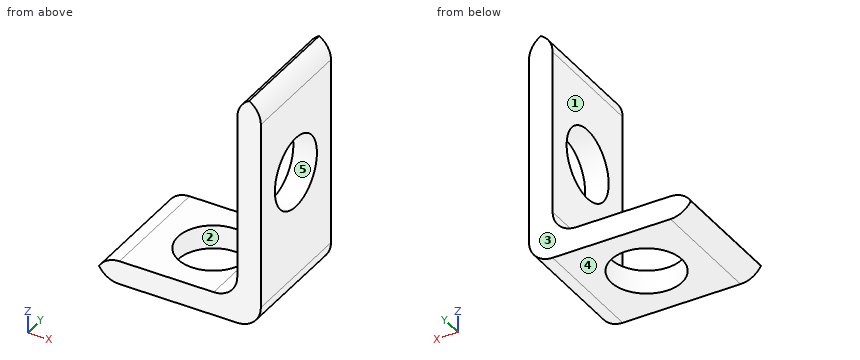
```python
from build123d import *

# Parameters (mm, degrees)
SKETCH1_W           = 7
SKETCH1_H           = 5
SKETCH1_R           = 1.5
BOSS_EXTRUDE1_DEPTH = 1
SKETCH2_W           = 1
SKETCH2_H           = 5
BOSS_EXTRUDE2_DEPTH = 9
SKETCH3_R           = 1.5
CUT_EXTRUDE1_DEPTH  = 1
FILLET1_R           = 1
FILLET2_R           = 1
FILLET3_R           = 1


# Some blends are built 0.0001 mm under size
with BuildPart() as part:
    # Sketch1 → Boss-Extrude1 (new body)
    with BuildSketch(Plane.XY):
        with Locations((3.5, 2.5)):
            Rectangle(SKETCH1_W, SKETCH1_H)
        with Locations((3.5, 2.5)):
            Circle(SKETCH1_R, mode=Mode.SUBTRACT)
    extrude(amount=BOSS_EXTRUDE1_DEPTH)

    # Sketch2 → Boss-Extrude2 (add)
    with BuildSketch(Plane.XY.offset(1)):
        with Locations((6.5, 2.5)):
            Rectangle(SKETCH2_W, SKETCH2_H)
    extrude(amount=BOSS_EXTRUDE2_DEPTH)

    # Sketch3 → Cut-Extrude1 (cut)
    with BuildSketch(Plane.ZY.offset(-6)):
        with Locations(Location((5.5, 2.5, 0), (0, 0, 270))):
            Circle(SKETCH3_R)
    extrude(amount=-CUT_EXTRUDE1_DEPTH, mode=Mode.SUBTRACT)

    # Fillet1
    fillet1_edges = [part.edges().sort_by_distance(p)[0] for p in [
        (6, 2.5, 1),
    ]]
    fillet(fillet1_edges, radius=FILLET1_R - 0.0001)  # a hair under: the kernel refuses the full size

    # Fillet2
    # the kernel refuses this fillet: 1 mm, written as the material it takes off along each edge
    with BuildSketch(Plane(origin=(7, -2.5, 10), x_dir=(-1, 0, 0), z_dir=(0, 1, 0)), Plane(origin=(0, 7.5, 0), x_dir=(0, 0, 1), z_dir=(0, -1, 0)), Plane(origin=(0, 7.5, 1), x_dir=(1, 0, 0), z_dir=(0, -1, 0))) as fillet2_piece_1:
        with BuildLine():
            CenterArc((FILLET2_R, -FILLET2_R), FILLET2_R, 90, 90)
            Line((0, -FILLET2_R), (0, 0))
            Line((0, 0), (FILLET2_R, 0))
        make_face()
    extrude(amount=10, mode=Mode.SUBTRACT)
    with BuildSketch(Plane(origin=(6, 7.5, 10), x_dir=(0, 0, -1), z_dir=(0, -1, 0))) as fillet2_piece_2:
        with BuildLine():
            CenterArc((FILLET2_R, FILLET2_R), FILLET2_R, 180, 90)
            Line((0, FILLET2_R), (0, 0))
            Line((0, 0), (FILLET2_R, 0))
        make_face()
    extrude(amount=10, mode=Mode.SUBTRACT)

    # Fillet3
    fillet3_edges = [part.edges().sort_by_distance(p)[0] for p in [
        (7, 2.5, 0),
    ]]
    fillet(fillet3_edges, radius=FILLET3_R)


solid = part.part
```
Build history of the part. All positions in model axes, mm. Face numbers are marked on the shaded views. A direction names the side the tool comes from. Round coordinates to 2 decimals unless told otherwise and drop trailing zeros. Loops run counter-clockwise (first coordinate to the right, second up) from the corner with the lowest first, then second, coordinate; pieces in that order, holes last. Notation, with made-up numbers: M -38.5,-3 L -15.5,-3 A25 cw -15.5,31 Z; hole C -11.75,62 d2. An arc over 180 degrees is marked long. Answer as CSV lines item,"result".
1. Cut at C-C on x = 3.5. Write the cut outline in (y, z).
Resolved:
outline,"M 0,0 L 1,0 L 1,1 L 0,1 Z; M 4,0 L 5,0 L 5,1 L 4,1 Z"
2. Cut at D-D on y = 0.8. Write the cut outline in (x, z).
Resolved:
outline,"M 0.13,0.5 A1 ccw 1,0 L 6,0 A1 ccw 7,1 L 7,9 A1 ccw 6.5,9.87 A1 ccw 6,9 L 6,2 A1 cw 5,1 L 1,1 A1 ccw Z"
3. Two-plate mould, pull along Y, no slides. Class the marked faces 3, 4 and 5: released by +Y, released by -Y, zero draft, split by the parting line, or undercut.
Resolved:
face 3,"released by +Y"
face 4,"zero draft"
face 5,"undercut"
4. Flat gauge pins, fed straight in: P1, Ø1.5, axis at y = 2.5, z = 8, coming from the -X side; P2, Ø1.8, axis at x = 3.5, y = 2.5, coming from the -Z side; P3, Ø3, axis at x = 5.5, z = 7, coming from the -Y side. Where does each tip first touch, or does it go through?
Resolved:
P1,"stops at x = 6"
P2,"passes through"
P3,"stops at y = 0"
5. Wall check: probe 1 along Y at (x, z) = (3.5, 0.7); probe 2 along X at (y, z) = (4.35, 3); probe 3 along Z at (x, y) = (1, 2.2). Give the ranges that are in metal, low to high. Write a range as [from, to].
Resolved:
probe 1,"y = [0, 1], [4, 5]"
probe 2,"x = [6, 7]"
probe 3,"z = [0, 1]"
6. 3-axis set-ups, long thin cutter, end or side, ignore diameter. For the marked faces 1 and 2: which of +Z, -Z, +X, -X, +Y, -Y reach the whole face in a straight line?
Resolved:
face 1,"+Z, -X, +Y, -Y"
face 2,"+Z, -Z"
7. Cut at A-A on z = 5.5. Write the cut outline in (x, y).
Resolved:
outline,"M 6,0 L 7,0 L 7,1 L 6,1 Z; M 6,4 L 7,4 L 7,5 L 6,5 Z"
8. Cut at B-B on y = 2.5. Count the separate pieces of the cut face and the enclosed holes in it, then the cut area to 3 significant figures.
Resolved:
separate pieces,"3"
enclosed holes,"0"
area,"9.23 mm²"
